```python
from build123d import *

# Parameters (mm, degrees)
SKETCH1_W                       = 63.5
SKETCH1_H                       = 24.13
BOSS_EXTRUDE1_DEPTH             = 4.064
BOSS_EXTRUDE2_REACH             = 36.207
BOSS_EXTRUDE2_DIRECTION_2_REACH = 36.207
CUT_EXTRUDE1_DEPTH              = 4.064
CUT_EXTRUDE1_DEPTH_BACK         = 66.752974943
SKETCH4_R                       = 8.636
FILLET1_R                       = 2.54
CUT_EXTRUDE2_DEPTH              = 73.348315655
BOSS_EXTRUDE3_DEPTH             = 2.54
BOSS_EXTRUDE4_START             = 2.54
BOSS_EXTRUDE4_DEPTH             = 2.54
BOSS_EXTRUDE5_DEPTH             = 3.81
CUT_EXTRUDE3_DEPTH              = 64.061052508
BOSS_EXTRUDE6_START             = -23.114
SKETCH12_W                      = 44.831
SKETCH12_H                      = 27.027043781
BOSS_EXTRUDE6_DEPTH             = 23.114
BOSS_EXTRUDE7_DEPTH             = 7.874
CUT_EXTRUDE4_START              = -6.219751
CUT_EXTRUDE4_DEPTH              = 6.219751
CUT_EXTRUDE5_DEPTH              = 27.027043781
SKETCH17_W                      = 6.9977
SKETCH17_H                      = 3.556
BOSS_EXTRUDE8_DEPTH             = 13.97
SKETCH18_W                      = 6.389869694
SKETCH18_H                      = 3.556
BOSS_EXTRUDE9_DEPTH             = 13.97
SKETCH19_W                      = 31.75
SKETCH19_H                      = 7.112
CUT_EXTRUDE6_DEPTH              = 13.97
CUT_EXTRUDE7_REACH              = 87.043
SKETCH20_R                      = 1.7145
FILLET2_R                       = 2.54
FILLET3_R                       = 2.54
FILLET4_R                       = 2.54
BOSS_EXTRUDE10_DEPTH            = 29.21
BOSS_EXTRUDE11_DEPTH            = 27.027043781
BOSS_EXTRUDE16_DEPTH            = 6.35
FILLET5_R                       = 6.35
FILLET6_R                       = 3.81


with BuildPart() as part:
    # Sketch1 → Boss-Extrude1 (new body)
    with BuildSketch(Plane(origin=(0, 0, 0), x_dir=(1, 0, 0), z_dir=(0, 1, 0))):
        Rectangle(SKETCH1_W, SKETCH1_H)
    extrude(amount=BOSS_EXTRUDE1_DEPTH)

    # Boss-Extrude2: up to this face of the body (flat: up to its plane)
    boss_extrude2_end = Plane(part.part.faces().sort_by_distance((0, 2.032, 12.065))[0])
    # Sketch2 → Boss-Extrude2 (add, up to the picked face)
    with BuildSketch(Plane.XY, mode=Mode.PRIVATE) as boss_extrude2_sk1:
        with BuildLine():
            Line((0, 4.064), (-26.716755185, 4.064))
            Line((-26.716755185, 4.064), (-31.571041118, 27.367716778))
            ThreePointArc((-31.571041118, 27.367716778), (-27.221246487, 47.076161415), (-11.87173913, 60.180974548))
            ThreePointArc((-11.87173913, 60.180974548), (-8.566242036, 58.774955714), (-9.97226087, 55.46945862))
            ThreePointArc((-9.97226087, 55.46945862), (-26.181898149, 25.654914521), (0, 4.064))
        make_face()
    boss_extrude2_tool1 = split(extrude(boss_extrude2_sk1.sketch, amount=BOSS_EXTRUDE2_REACH, mode=Mode.PRIVATE), bisect_by=boss_extrude2_end, keep=Keep.BOTH, mode=Mode.PRIVATE)
    add(boss_extrude2_tool1.solids().sort_by(Axis((-9.165723, 58.533271, 0), (0, 0, 1)))[0])

    # Boss-Extrude2 direction 2: up to this face of the body (flat: up to its plane)
    boss_extrude2_direction_2_end = Plane(part.part.faces().sort_by_distance((0, 2.032, -12.065))[0])
    # Sketch2 → Boss-Extrude2 direction 2 (add, up to the picked face)
    with BuildSketch(Plane.XY, mode=Mode.PRIVATE) as boss_extrude2_direction_2_sk1:
        with BuildLine():
            Line((0, 4.064), (-26.716755185, 4.064))
            Line((-26.716755185, 4.064), (-31.571041118, 27.367716778))
            ThreePointArc((-31.571041118, 27.367716778), (-27.221246487, 47.076161415), (-11.87173913, 60.180974548))
            ThreePointArc((-11.87173913, 60.180974548), (-8.566242036, 58.774955714), (-9.97226087, 55.46945862))
            ThreePointArc((-9.97226087, 55.46945862), (-26.181898149, 25.654914521), (0, 4.064))
        make_face()
    boss_extrude2_direction_2_tool1 = split(extrude(boss_extrude2_direction_2_sk1.sketch, amount=-BOSS_EXTRUDE2_DIRECTION_2_REACH, mode=Mode.PRIVATE), bisect_by=boss_extrude2_direction_2_end, keep=Keep.BOTH, mode=Mode.PRIVATE)
    add(boss_extrude2_direction_2_tool1.solids().sort_by(Axis((-9.165723, 58.533271, 0), (0, 0, -1)))[0])

    # Sketch4 → Cut-Extrude1 (cut, two sides: drawn at the far end of the back side and taken through both)
    with BuildSketch(Plane(origin=(0, 4.064, 0), x_dir=(1, 0, 0), z_dir=(0, 1, 0)).offset(-CUT_EXTRUDE1_DEPTH_BACK)):
        with Locations(Location((0, 0, 0), (0, 0, 270))):
            Circle(SKETCH4_R)
    extrude(amount=CUT_EXTRUDE1_DEPTH + CUT_EXTRUDE1_DEPTH_BACK, mode=Mode.SUBTRACT)

    # Fillet1
    fillet1_edges = [part.edges().sort_by_distance(p)[0] for p in [
        (-8.636, 5.50091846, 0),
        (8.636, 4.064, 0),
    ]]
    fillet(fillet1_edges, radius=FILLET1_R)

    # Sketch6 → Cut-Extrude2 (cut, through all)
    with BuildSketch(Plane.XY.offset(12.065)):
        Polygon((-31.75, 4.064), (-26.716755185, 4.064), (-25.870202757, 0), (-31.75, 0), align=None)
    extrude(amount=-CUT_EXTRUDE2_DEPTH, mode=Mode.SUBTRACT)

    # Sketch8 → Boss-Extrude3 (add)
    with BuildSketch(Plane.XY.offset(12.065)):
        with BuildLine():
            Line((31.75, 0), (31.75, 7.874))
            Line((31.75, 7.874), (-4.274632474, 7.874))
            ThreePointArc((-4.274632474, 7.874), (-23.508790492, 29.710248048), (-9.97226087, 55.46945862))
            ThreePointArc((-9.97226087, 55.46945862), (-8.566242036, 58.774955714), (-11.87173913, 60.180974548))
            ThreePointArc((-11.87173913, 60.180974548), (-27.221246487, 47.076161415), (-31.571041118, 27.367716778))
            Line((-31.571041118, 27.367716778), (-25.870202757, 0))
            Line((-25.870202757, 0), (31.75, 0))
        make_face()
    extrude(amount=BOSS_EXTRUDE3_DEPTH)

    # Sketch9 → Boss-Extrude4 (add)
    with BuildSketch(Plane(origin=(0, 0, -12.065), x_dir=(-1, 0, 0), z_dir=(0, 0, -1)).offset(BOSS_EXTRUDE4_START)):
        with BuildLine():
            Line((-31.75, 0), (-31.75, 7.874))
            Line((-31.75, 7.874), (4.274632474, 7.874))
            ThreePointArc((4.274632474, 7.874), (23.508790492, 29.710248048), (9.97226087, 55.46945862))
            ThreePointArc((9.97226087, 55.46945862), (8.566242036, 58.774955714), (11.87173913, 60.180974548))
            ThreePointArc((11.87173913, 60.180974548), (27.221246487, 47.076161415), (31.571041118, 27.367716778))
            Line((31.571041118, 27.367716778), (25.870202757, 0))
            Line((25.870202757, 0), (-31.75, 0))
        make_face()
    extrude(amount=-BOSS_EXTRUDE4_DEPTH)

    # Sketch10 → Boss-Extrude5 (add)
    with BuildSketch(Plane(origin=(0, 4.064, 0), x_dir=(1, 0, 0), z_dir=(0, 1, 0))):
        with BuildLine():
            Line((10.218295125, 14.605), (10.218295125, 12.065))
            ThreePointArc((10.218295125, 12.065), (22.283295125, 0), (10.218295125, -12.065))
            Line((10.218295125, -12.065), (10.218295125, -14.605))
            ThreePointArc((10.218295125, -14.605), (24.823295125, 0), (10.218295125, 14.605))
        make_face()
    extrude(amount=BOSS_EXTRUDE5_DEPTH)

    # Sketch11 → Cut-Extrude3 (cut, through all)
    with BuildSketch(Plane(origin=(0, 7.874, 0), x_dir=(1, 0, 0), z_dir=(0, 1, 0))):
        with BuildLine():
            Line((10.218295125, 14.605), (31.75, 14.605))
            Line((31.75, 14.605), (31.75, -14.605))
            Line((31.75, -14.605), (10.218295125, -14.605))
            ThreePointArc((10.218295125, -14.605), (24.823295125, 0), (10.218295125, 14.605))
        make_face()
    extrude(amount=-CUT_EXTRUDE3_DEPTH, mode=Mode.SUBTRACT)

    # Sketch12 → Boss-Extrude6 (add)
    with BuildSketch(Plane.XZ.offset(BOSS_EXTRUDE6_START)):
        with Locations((-8.8011, -28.11852189)):
            Rectangle(SKETCH12_W, SKETCH12_H)
    extrude(amount=BOSS_EXTRUDE6_DEPTH)

    # Sketch13 → Boss-Extrude7 (add)
    with BuildSketch(Plane.XZ):
        Polygon((10.218295125, -14.605), (13.6144, -14.605), (13.6144, -13.335525526), align=None)
    extrude(amount=-BOSS_EXTRUDE7_DEPTH)

    # Sketch14 → Cut-Extrude4 (cut)
    with BuildSketch(Plane.XY.offset(-14.605).offset(CUT_EXTRUDE4_START)):
        with BuildLine():
            Line((0, 13.017313502), (18.620278687, 13.017313502))
            Line((18.620278687, 13.017313502), (17.716686498, 30.734))
            ThreePointArc((17.716686498, 30.734), (-12.527589163, 43.261589163), (0, 13.017313502))
        make_face()
    extrude(amount=CUT_EXTRUDE4_DEPTH, mode=Mode.SUBTRACT)

    # Sketch16 → Cut-Extrude5 (cut)
    with BuildSketch(Plane.XY.offset(-14.605)):
        Polygon((-31.2166, 23.114), (-30.684969694, 23.114), (-25.870202757, 0), (-31.2166, 0), align=None)
    extrude(amount=-CUT_EXTRUDE5_DEPTH, mode=Mode.SUBTRACT)

    # Sketch17 → Boss-Extrude8 (add)
    with BuildSketch(Plane(origin=(0, 23.114, 0), x_dir=(1, 0, 0), z_dir=(0, 1, 0))):
        with Locations((10.11555, 34.413750632)):
            Rectangle(SKETCH17_W, SKETCH17_H)
    extrude(amount=BOSS_EXTRUDE8_DEPTH)

    # Sketch18 → Boss-Extrude9 (add)
    with BuildSketch(Plane(origin=(0, 23.114, 0), x_dir=(1, 0, 0), z_dir=(0, 1, 0))):
        with Locations((-27.490034847, 34.413750632)):
            Rectangle(SKETCH18_W, SKETCH18_H)
    extrude(amount=BOSS_EXTRUDE9_DEPTH)

    # Sketch19 → Cut-Extrude6 (cut)
    with BuildSketch(Plane(origin=(0, 37.084, 0), x_dir=(1, 0, 0), z_dir=(0, 1, 0))):
        with Locations((-8.8392, 36.191750632)):
            Rectangle(SKETCH19_W, SKETCH19_H)
    extrude(amount=-CUT_EXTRUDE6_DEPTH, mode=Mode.SUBTRACT)

    # Sketch20 → Cut-Extrude7 (cut, up to next)
    with BuildSketch(Plane(origin=(0, 0, -36.191750632), x_dir=(-1, 0, 0), z_dir=(0, 0, -1)), mode=Mode.PRIVATE) as cut_extrude7_sk1:
        with Locations((27.75585, 30.734)):
            Circle(SKETCH20_R)
    cut_extrude7_tool1 = extrude(cut_extrude7_sk1.sketch, amount=-CUT_EXTRUDE7_REACH, mode=Mode.PRIVATE) & part.part
    # Sketch20 → Cut-Extrude7 (cut, up to next)
    with BuildSketch(Plane(origin=(0, 0, -36.191750632), x_dir=(-1, 0, 0), z_dir=(0, 0, -1)), mode=Mode.PRIVATE) as cut_extrude7_sk2:
        with Locations((-10.11555, 30.734)):
            Circle(SKETCH20_R)
    cut_extrude7_tool2 = extrude(cut_extrude7_sk2.sketch, amount=-CUT_EXTRUDE7_REACH, mode=Mode.PRIVATE) & part.part
    add(cut_extrude7_tool1.solids().sort_by_distance((-27.75585, 30.734, -36.191751))[0], mode=Mode.SUBTRACT)
    add(cut_extrude7_tool2.solids().sort_by_distance((10.11555, 30.734, -36.191751))[0], mode=Mode.SUBTRACT)

    # Fillet2
    fillet2_edges = [part.edges().sort_by_distance(p)[0] for p in [
        (10.3251, 23.114, -36.191750632),
    ]]
    fillet(fillet2_edges, radius=FILLET2_R)

    # Fillet3
    fillet3_edges = [part.edges().sort_by_distance(p)[0] for p in [
        (-27.699584847, 23.114, -36.191750632),
    ]]
    fillet(fillet3_edges, radius=FILLET3_R)

    # Fillet4
    fillet4_edges = [part.edges().sort_by_distance(p)[0] for p in [
        (13.6144, 37.084, -34.413750632),
        (-30.684969694, 37.084, -34.413750632),
    ]]
    fillet(fillet4_edges, radius=FILLET4_R)

    # Sketch26 → Boss-Extrude10 (add)
    with BuildSketch(Plane.XY.offset(14.605)):
        Polygon((-25.870202757, 0), (-31.653563464, 0), (-31.571041118, 27.367716778), align=None)
    extrude(amount=-BOSS_EXTRUDE10_DEPTH)

    # Sketch22 → Boss-Extrude11 (add)
    with BuildSketch(Plane(origin=(0, 0, -14.605), x_dir=(-1, 0, 0), z_dir=(0, 0, -1))):
        Polygon((30.684969694, 23.114), (31.583867423, 23.114), (31.653563464, 0), (25.870202757, 0), align=None)
    extrude(amount=BOSS_EXTRUDE11_DEPTH)

    # Sketch23 → Boss-Extrude16 (add)
    with BuildSketch(Plane.XZ):
        with BuildLine():
            Line((-15.554631727, 14.605), (-44.353563464, 14.605))
            Line((-44.353563464, 14.605), (-44.353563464, -41.632043781))
            ThreePointArc((-44.353563464, -41.632043781), (-40.609144413, -50.636907459), (-31.583867423, -54.331852538))
            Line((-31.583867423, -54.331852538), (13.6144, -54.332043781))
            Line((13.6144, -54.332043781), (13.6144, -35.10352189))
            Line((13.6144, -35.10352189), (-15.554631727, -35.10352189))
            Line((-15.554631727, -35.10352189), (-15.554631727, 14.605))
        make_face()
        with BuildLine():
            Line((-34.701563464, 8.255), (-34.701563464, -42.545))
            ThreePointArc((-34.701563464, -42.545), (-38.003563464, -45.847), (-41.305563464, -42.545))
            Line((-41.305563464, -42.545), (-41.305563464, 8.255))
            ThreePointArc((-41.305563464, 8.255), (-38.003563464, 11.557), (-34.701563464, 8.255))
        make_face(mode=Mode.SUBTRACT)
        with BuildLine():
            Line((-24.859733712, -44.680043781), (6.890266288, -44.680043781))
            ThreePointArc((6.890266288, -44.680043781), (10.192266288, -47.982043781), (6.890266288, -51.284043781))
            Line((6.890266288, -51.284043781), (-24.859733712, -51.284043781))
            ThreePointArc((-24.859733712, -51.284043781), (-28.161733712, -47.982043781), (-24.859733712, -44.680043781))
        make_face(mode=Mode.SUBTRACT)
    extrude(amount=-BOSS_EXTRUDE16_DEPTH)

    # Fillet5
    fillet5_edges = [part.edges().sort_by_distance(p)[0] for p in [
        (13.6144, 3.175, -54.332043781),
        (-44.353563464, 3.175, 14.605),
    ]]
    fillet(fillet5_edges, radius=FILLET5_R)

    # Fillet6
    fillet6_edges = [part.edges().sort_by_distance(p)[0] for p in [
        (-31.609141812, 14.732, -41.632043781),
    ]]
    fillet(fillet6_edges, radius=FILLET6_R)


solid = part.part
```
The model under review builds one solid part; all positions refer to its coordinate system, in mm. A direction names the side the tool comes from. Coordinates: 2 decimals unless noted, no trailing zeros. Write each loop counter-clockwise with the first axis right and the second up, starting at its lowest first coordinate (ties: lowest second). Pieces come first, ordered by that corner, then holes. Notation, with made-up numbers: (49, 24) - (85, 24) arc R32 cw to (85, 54) - close; hole circle Ø2 at (-6.5, 74.25). An arc over 180 degrees is marked (long way). Answer in a Markdown table with one row per item. Add a question column.
Q1. To check wall thickness, follow line 1 along X through (y, z) = (0.95, 0); line 2 along Z through (x, y) = (0, 1) (3 decimals); line 3 along Y through (x, z) = (11, -39). State the ranges of each line that lie inside material, in increasing order. Write a range as from..to.
Q2. Consider section C-C on y = 46. Give the boundary of the cut face in (x, z) (3 decimals).
Q3. Consider section B-B on z = -31.5. Give the boundary of the cut face in (x, y), then the cut area to 3 significant figures.
Q4. Draft analysis for pull direction Y (two halves, no side actions). For faces 1 (the face through (-19, 17, 14.605)), 2 (the face through (22.1, 7.874, -3.2)), 3 (the face through (8.48, 31.25, -34.44)), state which applies: +Y half, -Y half, draft (parallel to the pull), parting line (faces both ways), or undercut.
Q5. Clearance check with flat-ended pins moving along their axes: pin 1 (1.8 mm diameter, centred on x = -26.5, y = 32.5, fed in from -Z); pin 2 (11 mm diameter, centred on x = -8.5, y = 18, fed in from +Z) (3 decimals); pin 3 (6 mm diameter, centred on x = -21.5, y = 33, fed in from +Z) (3 decimals); pin 4 (2 mm diameter, centred on x = 10.5, y = 33, fed in from +Z). State where each tip first meets the part, or that it passes through.
Q6. Consider section A-A on z = -19. Give the boundary of the cut face in (x, y), then the cut area to 3 significant figures.
Q7. Consider section D-D on x = 20.5. Give the boundary of the cut face in (y, z), then the cut area to 3 significant figures.
Q8. For faces 4 (the face through (-8.43, 1.01, -1.87)), 5 (the face through (-4, 13, -14.605)), 6 (the face through (13, 4.064, 0)), 7 (the face through (-30.685, 29, -34)), 8 (the face through (10, 33, -36.192)), list the 3-axis set-ups (+Z, -Z, +X, -X, +Y, -Y) from which the entire face can be reached by the end or side of a thin tool; tool diameter is ignored.
Answers below:
| question | item | result |
|---|---|---|
| 1 | line 1 | -44.35..-41.31, -34.7..-8.64, 8.64..24.82 |
| 1 | line 2 | -54.332..-51.284, -44.68..-8.636, 8.636..14.605 |
| 1 | line 3 | 0..23.11 |
| 2 | outline | (-27.839, -14.605) - (-20.01, -14.605) - (-20.01, -12.065) - (-21.869, -12.065) - (-21.869, 12.065) - (-20.01, 12.065) - (-20.01, 14.605) - (-27.839, 14.605) - close |
| 3 | outline | (-44.35, 0) - (-41.31, 0) - (-41.31, 6.35) - (-44.35, 6.35) - close; (-34.7, 0) - (13.61, 0) - (13.61, 23.11) - (-31.58, 23.11) - (-31.63, 6.35) - (-34.7, 6.35) - close |
| 3 | area | 1,080 mm² |
| 4 | face 1 | draft |
| 4 | face 2 | +Y half |
| 4 | face 3 | undercut |
| 5 | pin 1 | z = -36.19 |
| 5 | pin 2 | z = -14.605 |
| 5 | pin 3 | z = 14.605 |
| 5 | pin 4 | z = -32.64 |
| 6 | outline | (-44.35, 0) - (-41.31, 0) - (-41.31, 6.35) - (-44.35, 6.35) - close; (-34.7, 0) - (13.61, 0) - (13.61, 13.02) - (0, 13.02) arc R17.72 cw to (-15.99, 23.11) - (-31.58, 23.11) - (-31.63, 6.35) - (-34.7, 6.35) - close |
| 6 | area | 831 mm² |
| 7 | outline | (0, -10.37) - (7.87, -10.37) - (7.87, -6.31) - (4.06, -6.31) - (4.06, 6.31) - (7.87, 6.31) - (7.87, 10.37) - (0, 10.37) - close |
| 7 | area | 115 mm² |
| 8 | face 4 | -Y |
| 8 | face 5 | +Z, +X |
| 8 | face 6 | +Y |
| 8 | face 7 | -Z, -X, +Y |
| 8 | face 8 | -Z, +X, -X, +Y |
